from build123d import *

# Parameters (mm, degrees)
F0_R     = 1.5
F0_R_2   = 15
F1_DEPTH = 15
F2_W     = 10
F2_H     = 10
F3_DEPTH = 15
F4_W     = 10
F4_H     = 10
F5_DEPTH = 15
F6_W     = 10
F6_H     = 10
F7_DEPTH = 15
F8_R     = 9.99999


# Not quite as in the source:
# - a fillet or chamfer is up to 0.001 mm smaller than in the source, because OpenCascade refuses the exact size


with BuildPart() as f1:
    # F0 (on Top) → F1 (new body)
    with BuildSketch(Plane.XY):
        Polygon((-24.3407530135, 22.4126278684), (-31.5135795584, 9.2387689289), (-22.7389262459, 4.1727204769), (-37.7220713048, -21.7788480222), (-7.5, -21.7788480222), (-7.5, -31.7788480222), (0, -31.7788480222), (7.5, -31.7788480222), (7.5, -21.7788480222), (37.7220713048, -21.7788480222), (22.8180813967, 4.0356197342), (31.4860692862, 9.0400848755), (24.5212116355, 22.3250672958), (14.9900065464, 16.8222234719), (-0.6591394661, 43.9273394607), (-15.1098627306, 17.3866460996), align=None)
        with Locations((0, -21.7788480222)):
            Circle(F0_R, mode=Mode.SUBTRACT)
        Circle(F0_R_2, mode=Mode.SUBTRACT)
        with Locations((-18.8610356524, 10.8894240111)):
            Circle(F0_R, mode=Mode.SUBTRACT)
        with Locations((18.8610356524, 10.8894240111)):
            Circle(F0_R, mode=Mode.SUBTRACT)
    extrude(amount=F1_DEPTH)

    # F2 (on face) → F3 (cut)
    with BuildSketch(Plane.XZ.offset(31.7788480222)):
        with Locations((0, 7.5)):
            Rectangle(F2_W, F2_H)
    extrude(amount=-F3_DEPTH, mode=Mode.SUBTRACT)

    # F4 (on face) → F5 (cut)
    with BuildSketch(Plane(origin=(-28.1875812899, 15.3474112818, 0), x_dir=(-0.4781884363, -0.8782572626, 0), z_dir=(-0.8782572626, 0.4781884363, 0))):
        with Locations((0, 7.5)):
            Rectangle(F4_W, F4_H)
    extrude(amount=-F5_DEPTH, mode=Mode.SUBTRACT)

    # F6 (on face) → F7 (cut)
    with BuildSketch(Plane(origin=(28.415383594, 14.8972046453, 0), x_dir=(-0.4643238434, 0.8856654947, 0), z_dir=(0.8856654947, 0.4643238434, 0))):
        with Locations((0.8867585393, 7.5)):
            Rectangle(F6_W, F6_H)
    extrude(amount=-F7_DEPTH, mode=Mode.SUBTRACT)

    # F8 (radius 10 in the source; OpenCascade refuses exactly that, so slightly less here)
    f8_edges = [f1.edges().sort_by_distance(p)[0] for p in [
        (37.722071, -21.778848, 7.5),
        (-0.659139, 43.927339, 7.5),
        (14.990007, 16.822223, 7.5),
        (22.818081, 4.03562, 7.5),
        (7.5, -21.778848, 7.5),
        (-7.5, -21.778848, 7.5),
        (-37.722071, -21.778848, 7.5),
        (-22.738926, 4.17272, 7.5),
        (-15.109863, 17.386646, 7.5),
    ]]
    fillet(f8_edges, radius=F8_R)


solid = f1.part
Verification items for the finished model (mm, model axes). A direction names the side the tool comes from. Coordinates: 2 decimals unless noted, no trailing zeros. Order: outer loops, then holes, each group sorted by start corner. A loop starts at its lowest first (then second) coordinate and runs counter-clockwise, first axis right, second up.
Item 1: Access from +Z, -Z, +X, -X, +Y, -Y to the whole of each face (thin tool, end or side, straight path). Record for faces 1 (the face through (26.85, 3.07, 7.6)), 2 (the face through (0, -16.779, 8)), 3 (the face through (-26.77, 3.21, 7.6)), 4 (the face through (-19.3, 16.2, 7.4)), 5 (the face through (-22, 12, 12.5)).
Filled in:
face 1: +Z, -Z, +X
face 2: -Y
face 3: +Z, -Z, -X
face 4: -X
face 5: none
Item 2: Material ranges on L1, parallel to Y at x = 0, z = 14.1; L2, parallel to Y at x = 0, z = 9.5; L3, parallel to X at y = 22, z = 6.25, recorded low to high.
Filled in:
L1: y = -31.78 to -23.28, -20.28 to -15, 15 to 33.48
L2: y = -16.78 to -15, 15 to 33.48
L3: x = -24.57 to -23.57, -14.65 to 13.35, 23.96 to 24.69
Item 3: Section check B-B, the plane x = -3. Enter the section's corners in (y, z), then the cut area to 3 significant figures.
Filled in:
outline: (-31.78, 0) - (-14.7, 0) - (-14.7, 15) - (-31.78, 15) - (-31.78, 12.5) - (-16.78, 12.5) - (-16.78, 2.5) - (-31.78, 2.5) - close; (14.7, 0) - (33.14, 0) - (33.14, 15) - (14.7, 15) - close
area: 383 mm2
Item 4: Section check C-C, the plane y = -8. Enter the section's corners in (x, z), then the cut area to 3 significant figures.
Filled in:
outline: (-29.66, 0) - (-12.69, 0) - (-12.69, 15) - (-29.66, 15) - close; (12.69, 0) - (29.66, 0) - (29.66, 15) - (12.69, 15) - close
area: 509 mm2
Item 5: Release check for a two-part mould opening along X. For faces 6 (the face through (-25.486, 20.309, 7.395)), 7 (the face through (19, -21.779, 7)), 8 (the face through (0, -24, 2.5)) record: +X half, -X half, draft (parallel to the pull), parting line (faces both ways), or undercut.
Filled in:
face 6: -X half
face 7: draft
face 8: undercut
Item 6: Section check A-A, the plane y = 0. Enter the section's corners in (x, z), then the cut area to 3 significant figures.
Filled in:
outline: (-26.41, 0) - (-15, 0) - (-15, 15) - (-26.41, 15) - close; (15, 0) - (26.49, 0) - (26.49, 15) - (15, 15) - close
area: 343 mm2
Item 7: Depth check by flat-ended pin: pin 1 (5 mm diameter, centred on x = 3, y = 26.5, fed in from -Z); pin 2 (8 mm diameter, centred on y = 26.5, z = 6.5, fed in from -X); pin 3 (2.5 mm diameter, centred on x = -19, z = 7.5, fed in from -Y); pin 4 (1 mm diameter, centred on x = -11.5, y = 6, fed in from +Z) (3 decimals). Enter the tip coordinate at first touch or a pass-through.
Filled in:
pin 1: stops at z = 0
pin 2: stops at x = -13.76
pin 3: stops at y = -21.78
pin 4: passes through
